Solid Edge part; units mm, degrees
sketch "Sketch1" plane through (0, 0, 0) normal (0, -1, 0) x (1, 0, 0)
  circle A0 centre (75, 0) radius 2.5
  line L0 (-75.3333, 4.9889) -> (-0.6667, 9.9778)
  line L1 (0.6667, 9.9778) -> (75.3333, 4.9889)
  line L2 (75.3333, -4.9889) -> (0.6667, -9.9778)
  arc A1 (0.6667, -9.9778) -> (-0.6667, -9.9778) centre (0, 0) cw
  line L3 (-0.6667, -9.9778) -> (-75.3333, -4.9889)
  arc A2 (-75.3333, -4.9889) -> (-75.3333, 4.9889) centre (-75, 0) cw
  arc A3 (-0.6667, 9.9778) -> (0.6667, 9.9778) centre (0, 0) cw
  arc A4 (75.3333, 4.9889) -> (75.3333, -4.9889) centre (75, 0) cw
  circle A5 centre (0, 0) radius 2.5
  circle A6 centre (-75, 0) radius 2.5
extrude "Protrusion1" add sketch "Sketch1" along normal mid plane 10
Design review of the part built by this model. Coordinates are the model's own, in mm. Coordinates: 2 decimals unless noted, no trailing zeros. Order: outer loops, then holes, each group sorted by start corner. A loop starts at its lowest first (then second) coordinate and runs counter-clockwise, first axis right, second up. Notation, with made-up numbers: (71, 76.5) - (107, 76.5) arc R8 ccw to (107, 83.5) - close; hole circle Ø7 at (30, -30.5). An arc over 180 degrees is marked (long way). Put each result on its own line as item: value.
1) Take a section at A-A, the plane z = 0. Give the boundary of the cut face in (x, y), and give its area (3 significant figures).
Response values:
outline: (-80, -5) - (-77.5, -5) - (-77.5, 5) - (-80, 5) - close; (-72.5, -5) - (-2.5, -5) - (-2.5, 5) - (-72.5, 5) - close; (2.5, -5) - (72.5, -5) - (72.5, 5) - (2.5, 5) - close; (77.5, -5) - (80, -5) - (80, 5) - (77.5, 5) - close
area: 1,450 mm²
2) Insertion check: P1, Ø1, axis at x = -22.5, y = 3, coming from the +Z side; P2, Ø2, axis at y = -2, z = -5, coming from the -X side; P3, Ø2, axis at y = -2, z = -2.5, coming from the -X side; P4, Ø4.5, axis at x = 0, z = 0, coming from the +Y side. Each pin has a flat end and moves straight along its axis. Give the tip position at first contact, or say it passes through.
Response values:
P1: stops at z = 8.55
P2: stops at x = -78
P3: stops at x = -79.77
P4: passes through
3) Take a section at B-B, the plane y = 0.75. Give the boundary of the cut face in (x, z), and give its area (3 significant figures).
Response values:
outline: (-75.33, -4.99) - (-0.67, -9.98) arc R10 ccw to (0.67, -9.98) - (75.33, -4.99) arc R5 ccw to (75.33, 4.99) - (0.67, 9.98) arc R10 ccw to (-0.67, 9.98) - (-75.33, 4.99) arc R5 ccw to start; hole circle Ø5 at (-75, 0); hole circle Ø5 at (0, 0); hole circle Ø5 at (75, 0)
area: 2,270 mm²
4) Take a section at D-D, the plane z = -7.5. Give the boundary of the cut face in (x, y), and give its area (3 significant figures).
Response values:
outline: (-37.75, -5) - (37.75, -5) - (37.75, 5) - (-37.75, 5) - close
area: 755 mm²
5) Wall thickness on L1, parallel to Z at x = 75, y = 2.5; L2, parallel to Z at x = 0, y = -0.5; L3, parallel to Z at x = 11.5, y = -4.25: over which ranges is each line inside the solid? List them lowest first. Write a range as from..to.
Response values:
L1: z = -5.01..-2.5, 2.5..5.01
L2: z = -10..-2.5, 2.5..10
L3: z = -9.25..9.25
6) Take a section at C-C, the plane x = 29. Give the boundary of the cut face in (y, z), and give its area (3 significant figures).
Response values:
outline: (-5, -8.08) - (5, -8.08) - (5, 8.08) - (-5, 8.08) - close
area: 162 mm²
7) The part is to be moulded in two halves that separate along X. For faces 1 (the face through (-80, 0, 0)), 2 (the face through (80, 0, 0)), 3 (the face through (72.5, 0.1, -0.1)), say which applies: released by +X, released by -X, zero draft, split by the parting line, or undercut.
Response values:
face 1: released by -X
face 2: released by +X
face 3: undercut
